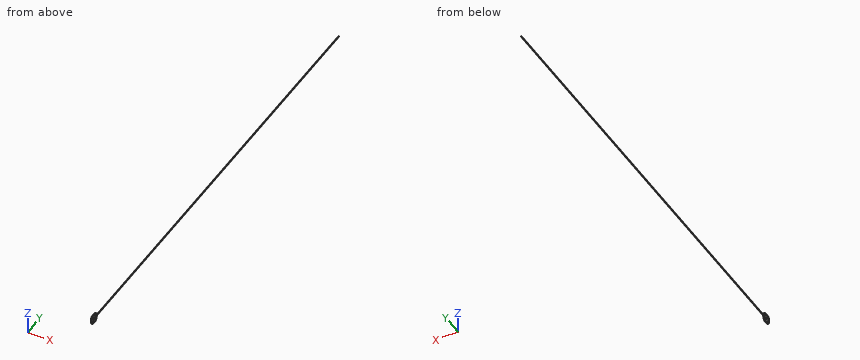
Autodesk Inventor part; units mm, degrees
ref_plane "YZ Plane" through (0, 0, 0) normal (1, 0, 0) x (0, 1, 0)
ref_plane "XZ Plane" through (0, 0, 0) normal (0, 1, 0) x (-1, 0, 0)
ref_plane "XY Plane" through (0, 0, 0) normal (0, 0, 1) x (1, 0, 0)
sketch "Sketch1" plane through (0, 0, 0) normal (0, 1, 0) x (-1, 0, 0)
  circle A0 centre (0, 0) radius 1
  dimension "d0" = 2
extrude "Extrusion1" add sketch "Sketch1" along normal blind 1200
sketch "Sketch2" plane through (0, 0, 0) normal (0, -1, 0) x (1, 0, 0)
  line L0 (-1, -12.5) -> (1, -12.5)
  line L1 (1, -12.5) -> (1, 12.5)
  line L2 (1, 12.5) -> (-1, 12.5)
  line L3 (-1, 12.5) -> (-1, -12.5)
  line L4 (-1, -12.5) -> (1, 12.5) construction
  line L5 (1, -12.5) -> (-1, 12.5) construction
  point P0 (0, 0)
  dimension "d3" = 2
  dimension "d4" = 25
extrude "Extrusion2" add sketch "Sketch2" against normal blind 25
fillet "Fillet1" radius 10 4 edges at (0, 25, 12.5) (0, 25, -12.5) (0, 0, 12.5) (0, 0, -12.5)
sketch "Sketch3" plane through (-1, 0, -2.5) normal (-1, 0, 0) x (0, 0, 1)
  circle A0 centre (2.5, 12.5) radius 3
  point P0 (2.5, 0)
  dimension "d8" = 6
hole "Hole1" at (-1, 12.5, 0) direction (1, 0, 0) diameter 6 end through all
sketch "Sketch4" plane through (1, 0, 2.5) normal (1, 0, 0) x (0, 0, -1)
  circle A0 centre (8.1569, 18.1569) radius 1.8
  circle A1 centre (8.1569, 6.8431) radius 1.8
  circle A2 centre (-3.1569, 6.8431) radius 1.8
  circle A3 centre (-3.1569, 18.1569) radius 1.8
  point P0 (2.5, 0)
hole "Hole2" at (1, 18.1569, -5.6569) at (1, 6.8431, -5.6569) at (1, 6.8431, 5.6569) at (1, 18.1569, 5.6569) direction (-1, 0, 0) diameter 4 end through all
properties part number "Hook Whip"
Can you work these out from the model? Positions are in its coordinate system, mm. Give positions to 0.01 mm unless a question says otherwise; leave off trailing zeros. Order: outer loops, then holes, each group sorted by start corner. A loop starts at its lowest first (then second) coordinate and runs counter-clockwise, first axis right, second up. Notation, with made-up numbers: M 59,81.5 L 65,81.5 A23 cw 65,117.5 Z; hole C 81,51 d10. An arc over 180 degrees is marked long. Use a Markdown table: item, result. Add a question column.
Item 1: Suppose I cut it at A-A (x = 0.7). List the corners of the cut face in (y, z) for me.
Item 2: If I drill on L1, parallel to Y at x = 0.55, z = 1.75; L2, parallel to Y at x = 0.6, z = -5.5; L3, parallel to Y at x = -0.6, z = -0.75, over which ranges is the centre line in solid material (lowest first)? Write a range as [from, to].
Item 3: Suppose I cut it at B-B (y = 372.5). List the corners of the cut face in (x, z) for me, then the cut area to 3 significant figures.
Answer sheet:
| question | item | result |
|---|---|---|
| 1 | outline | M 0,-2.5 A10 ccw 10,-12.5 L 15,-12.5 A10 ccw 25,-2.5 L 25,-0.71 L 1200,-0.71 L 1200,0.71 L 25,0.71 L 25,2.5 A10 ccw 15,12.5 L 10,12.5 A10 ccw 0,2.5 Z; hole C 6.84,-5.66 d4; hole C 6.84,5.66 d4; hole C 12.5,0 d6; hole C 18.16,-5.66 d4; hole C 18.16,5.66 d4 |
| 2 | L1 | y = [0, 10.06], [14.94, 25] |
| 2 | L2 | y = [0.46, 4.85], [8.84, 16.16], [20.15, 24.54] |
| 2 | L3 | y = [0, 9.6], [15.4, 1200] |
| 3 | outline | C 0,0 d2 |
| 3 | area | 3.14 mm² |
